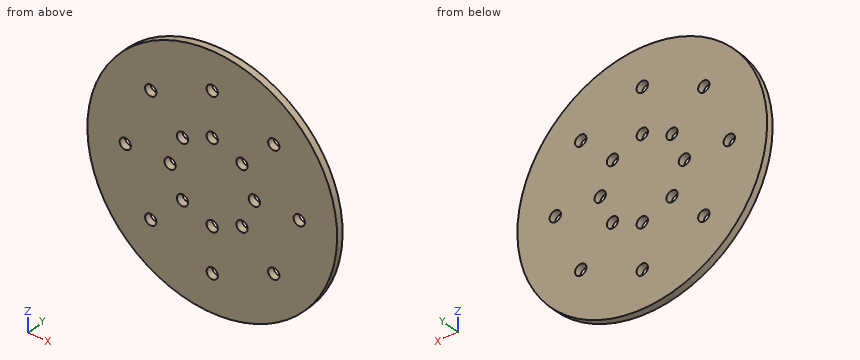
```python
from build123d import *

# Parameters (mm, degrees)
SKETCH1_R               = 56.5
SKETCH1_R_2             = 2.5527
BOSS_EXTRUDE1_DEPTH     = 3.175
F_1_4_20_TAPPED_HOLE1_D = 5.1054


with BuildPart() as part:
    # Sketch1 → Boss-Extrude1 (new body)
    # profile 1 of 9: a face of its own
    with BuildSketch(Plane(origin=(0, 0, 0), x_dir=(1, 0, 0), z_dir=(0, 1, 0))):
        with Locations(Location((0, 0, 0), (0, 0, 270))):
            Circle(SKETCH1_R)
        with Locations((-13.470384182, 13.470384182)):
            Circle(SKETCH1_R_2, mode=Mode.SUBTRACT)
        with Locations((-19.05, 0)):
            Circle(SKETCH1_R_2, mode=Mode.SUBTRACT)
        with Locations((-13.470384182, -13.470384182)):
            Circle(SKETCH1_R_2, mode=Mode.SUBTRACT)
        with Locations((0, -19.05)):
            Circle(SKETCH1_R_2, mode=Mode.SUBTRACT)
        with Locations((13.470384182, -13.470384182)):
            Circle(SKETCH1_R_2, mode=Mode.SUBTRACT)
        with Locations((19.05, 0)):
            Circle(SKETCH1_R_2, mode=Mode.SUBTRACT)
        with Locations((13.470384182, 13.470384182)):
            Circle(SKETCH1_R_2, mode=Mode.SUBTRACT)
        with Locations((0, 19.05)):
            Circle(SKETCH1_R_2, mode=Mode.SUBTRACT)
    # profile 2 of 9: a face of its own
    with BuildSketch(Plane(origin=(0, 0, 0), x_dir=(1, 0, 0), z_dir=(0, 1, 0))):
        with Locations((13.470384182, 13.470384182)):
            Circle(SKETCH1_R_2)
    # profile 3 of 9: a face of its own
    with BuildSketch(Plane(origin=(0, 0, 0), x_dir=(1, 0, 0), z_dir=(0, 1, 0))):
        with Locations((0, 19.05)):
            Circle(SKETCH1_R_2)
    # profile 4 of 9: a face of its own
    with BuildSketch(Plane(origin=(0, 0, 0), x_dir=(1, 0, 0), z_dir=(0, 1, 0))):
        with Locations((19.05, 0)):
            Circle(SKETCH1_R_2)
    # profile 5 of 9: a face of its own
    with BuildSketch(Plane(origin=(0, 0, 0), x_dir=(1, 0, 0), z_dir=(0, 1, 0))):
        with Locations((13.470384182, -13.470384182)):
            Circle(SKETCH1_R_2)
    # profile 6 of 9: a face of its own
    with BuildSketch(Plane(origin=(0, 0, 0), x_dir=(1, 0, 0), z_dir=(0, 1, 0))):
        with Locations((0, -19.05)):
            Circle(SKETCH1_R_2)
    # profile 7 of 9: a face of its own
    with BuildSketch(Plane(origin=(0, 0, 0), x_dir=(1, 0, 0), z_dir=(0, 1, 0))):
        with Locations((-13.470384182, -13.470384182)):
            Circle(SKETCH1_R_2)
    # profile 8 of 9: a face of its own
    with BuildSketch(Plane(origin=(0, 0, 0), x_dir=(1, 0, 0), z_dir=(0, 1, 0))):
        with Locations((-13.470384182, 13.470384182)):
            Circle(SKETCH1_R_2)
    # profile 9 of 9: a face of its own
    with BuildSketch(Plane(origin=(0, 0, 0), x_dir=(1, 0, 0), z_dir=(0, 1, 0))):
        with Locations((-19.05, 0)):
            Circle(SKETCH1_R_2)
    extrude(amount=BOSS_EXTRUDE1_DEPTH)

    # 1/4-20 Tapped Hole1 (through all)
    with Locations(Plane(origin=(13.470384182, 0, -13.470384182), x_dir=(0, 0, -1), z_dir=(0, -1, 0))):
        with Locations((0, 0), (-13.470384182, 5.579615818), (-26.940768364, 0), (-32.520384182, -13.470384182), (-26.940768364, -26.940768364), (-13.470384182, -32.520384182), (0, -26.940768364), (5.579615818, -13.470384182), (25.899615818, -13.470384182), (14.368409793, -41.309178157), (-13.470384182, -52.840384182), (-41.309178157, -41.309178157), (-52.840384182, -13.470384182), (-41.309178157, 14.368409793), (-13.470384182, 25.899615818), (14.368409793, 14.368409793)):
            Hole(F_1_4_20_TAPPED_HOLE1_D / 2)


solid = part.part
```
For this review, take the finished solid that the model builds, in its own axes (mm). Give positions to 0.01 mm unless a question says otherwise; leave off trailing zeros. Order: outer loops, then holes, each group sorted by start corner. A loop starts at its lowest first (then second) coordinate and runs counter-clockwise, first axis right, second up.
1) Take a section at D-D (x = 19.05). Give the boundary of the cut face in (y, z) (3 decimals), then the cut area to 3 significant figures.
2) Take a section at A-A (z = 0). Give the boundary of the cut face in (x, y) (3 decimals), then the cut area to 3 significant figures.
3) Take a section at C-C (y = 0.65). State how many separate pieces and enclosed holes the cut face has, then the cut area to 3 significant figures.
4) Take a section at B-B (z = 19.05). Give the boundary of the cut face in (x, y) (3 decimals), then the cut area to 3 significant figures.
5) Insertion check: pin 1 (6.5 mm diameter, centred on x = -13.47, z = -13.47, fed in from -Y); pin 2 (1.5 mm diameter, centred on x = -33, y = 1, fed in from +Z); pin 3 (1.5 mm diameter, centred on y = 0.5, z = -10, fed in from +X). Each pin has a flat end and moves straight along its axis. Give the tip position at first contact, or say it passes through.
6) Wall thickness on line 1 (X direction, y = 1.75, z = -28.5); line 2 (Z direction, x = -27.5, y = 2.25); line 3 (Z direction, x = 13, y = 0.35): over which ranges is each line inside the solid? List them lowest first.
Derived:
1. outline: (0, -53.192) - (3.175, -53.192) - (3.175, -2.553) - (0, -2.553) - close; (0, 2.553) - (3.175, 2.553) - (3.175, 53.192) - (0, 53.192) - close
1. area: 322 mm2
2. outline: (-56.5, 0) - (-41.923, 0) - (-41.923, 3.175) - (-56.5, 3.175) - close; (-36.817, 0) - (-21.603, 0) - (-21.603, 3.175) - (-36.817, 3.175) - close; (-16.497, 0) - (16.497, 0) - (16.497, 3.175) - (-16.497, 3.175) - close; (21.603, 0) - (36.817, 0) - (36.817, 3.175) - (21.603, 3.175) - close; (41.923, 0) - (56.5, 0) - (56.5, 3.175) - (41.923, 3.175) - close
2. area: 294 mm2
3. separate pieces: 1
3. enclosed holes: 16
3. area: 9,700 mm2
4. outline: (-53.192, 0) - (-2.553, 0) - (-2.553, 3.175) - (-53.192, 3.175) - close; (2.553, 0) - (53.192, 0) - (53.192, 3.175) - (2.553, 3.175) - close
4. area: 322 mm2
5. pin 1: stops at y = 0
5. pin 2: stops at z = 46.39
5. pin 3: stops at x = 55.74
6. line 1: x = -48.79 to -30.3, -25.37 to 25.37, 30.3 to 48.79
6. line 2: z = -49.36 to -30.37, -25.31 to 25.31, 30.37 to 49.36
6. line 3: z = -54.98 to -15.98, -10.96 to 10.96, 15.98 to 54.98
